Autodesk Inventor part; units mm, degrees
ref_plane "YZ Plane" through (0, 0, 0) normal (1, 0, 0) x (0, 1, 0)
ref_plane "XZ Plane" through (0, 0, 0) normal (0, 1, 0) x (-1, 0, 0)
ref_plane "XY Plane" through (0, 0, 0) normal (0, 0, 1) x (1, 0, 0)
sketch "Skizze1" plane through (0, 0, 0) normal (0, 0, 1) x (1, 0, 0)
  line L0 (-4.5, 3.25) -> (-4.5, 2.25)
  arc A0 (-3.564, 1.602) -> (-4.5, 2.25) centre (-4.5, 1.25) ccw
  line L1 (-3.564, 1.602) -> (-3.2351, 1.602)
  line L2 (-3.2351, 1.602) -> (-3.2351, 0.898)
  line L3 (-3.2351, 0.898) -> (-3.564, 0.898)
  arc A1 (-4.5, 0.25) -> (-3.564, 0.898) centre (-4.5, 1.25) ccw
  line L4 (-4.5, 0.25) -> (-4.5, -3.25)
  line L5 (-4.5, -3.25) -> (4.5, -3.25)
  line L6 (4.5, -3.25) -> (4.5, 0.25)
  arc A2 (3.564, 0.898) -> (4.5, 0.25) centre (4.5, 1.25) ccw
  line L7 (3.564, 0.898) -> (3.2351, 0.898)
  line L8 (3.2351, 0.898) -> (3.2351, 1.602)
  line L9 (3.2351, 1.602) -> (3.564, 1.602)
  arc A3 (4.5, 2.25) -> (3.564, 1.602) centre (4.5, 1.25) ccw
  line L10 (4.5, 2.25) -> (4.5, 3.25)
  line L11 (4.5, 3.25) -> (-4.5, 3.25)
  line L12 (4.575, -3.325) -> (-4.575, -3.325)
  line L13 (-4.575, -3.325) -> (-4.575, 0.328)
  arc A4 (-4.575, 0.328) -> (-3.6174, 0.973) centre (-4.5, 1.25) ccw
  line L14 (-3.6174, 0.973) -> (-3.3101, 0.973)
  line L15 (-3.3101, 0.973) -> (-3.3101, 1.527)
  line L16 (-3.3101, 1.527) -> (-3.6174, 1.527)
  arc A5 (-3.6174, 1.527) -> (-4.575, 2.172) centre (-4.5, 1.25) ccw
  line L17 (-4.575, 2.172) -> (-4.575, 3.325)
  line L18 (-4.575, 3.325) -> (4.575, 3.325)
  line L19 (4.575, 3.325) -> (4.575, 2.172)
  arc A6 (4.575, 2.172) -> (3.6174, 1.527) centre (4.5, 1.25) ccw
  line L20 (3.6174, 1.527) -> (3.3101, 1.527)
  line L21 (3.3101, 1.527) -> (3.3101, 0.973)
  line L22 (3.3101, 0.973) -> (3.6174, 0.973)
  arc A7 (3.6174, 0.973) -> (4.575, 0.328) centre (4.5, 1.25) ccw
  line L23 (4.575, 0.328) -> (4.575, -3.325)
  circle A8 centre (-15.1, -13.35) radius 3.5
  line L24 (-20.2, -17.25) -> (-22.2, -15.25)
  line L25 (-20.2, -17.25) -> (9.8, -17.25)
  line L26 (9.8, -17.25) -> (9.8, 6.75)
  line L27 (-11.8, 6.75) -> (9.8, 6.75)
  line L28 (-11.8, 11.75) -> (-11.8, 6.75)
  line L29 (-20.2, 11.75) -> (-11.8, 11.75)
  line L30 (-22.2, 9.75) -> (-20.2, 11.75)
  line L31 (-22.2, -15.25) -> (-22.2, 9.75)
  line L32 (-11.8, 6.75) -> (-9.8, 6.75)
  line L33 (-9.8, 6.75) -> (-9.8, 11.75)
  line L34 (-9.8, 11.75) -> (-11.8, 11.75)
  line L35 (-11.8, 11.75) -> (-11.8, 6.75)
  line L36 (9.8, 11.75) -> (-20.2, 11.75)
  circle A9 centre (-15.1, -13.35) radius 1.1
  line L37 (-22.2, -15.25) -> (-20.2, -17.25)
  line L38 (-22.2, -15.25) -> (-22.2, 9.75)
  line L39 (-20.2, 11.75) -> (-22.2, 9.75)
  line L40 (9.8, 11.75) -> (-20.2, 11.75)
  line L41 (9.8, -17.25) -> (9.8, 11.75)
  line L42 (9.8, -17.25) -> (-20.2, -17.25)
  line L43 (-10, 6.75) -> (10, 6.75)
  line L44 (10, 6.75) -> (10, -6.75)
  line L45 (10, -6.75) -> (-10, -6.75)
  line L46 (-10, -6.75) -> (-10, 6.75)
  line L47 (-10, 6.75) -> (10, -6.75) construction
  line L48 (10, 6.75) -> (-10, -6.75) construction
  line L49 (10, 6.75) -> (-10, 6.75)
  line L50 (-10, 6.75) -> (-10, 11.75)
  line L51 (-10, 11.75) -> (10, 11.75)
  line L52 (10, 11.75) -> (10, 6.75)
  line L53 (-4.575, 0.328) -> (-4.575, 2.172)
  line L54 (4.575, 0.328) -> (4.575, 2.172)
  line L55 (9.8, 11.75) -> (-20.2, 11.75)
  point P0 (0, 0)
  point P1 (4.5, -1.5)
  point P2 (4.575, -1.4985)
  dimension "d0" = 0.075
  dimension "d1" = 20
  dimension "d2" = 13.5
extrude "Extrusion1" add sketch "Skizze1" along normal blind 25 contours L45 L46 L27 L26 | L26 L43 L44 L45 | L27 L33 L36 L41 | L41 L51 L52 L43 | L27 L50 L34 L33
sketch "Skizze2" plane through (-10, 11.75, 0) normal (0, 1, 0) x (1, 0, 0)
  line L0 (20, 0) -> (0, 0)
  line L1 (0, 0) -> (0, -25)
  line L2 (20, -25) -> (0, -25)
  line L3 (20, 0) -> (20, -25)
  line L4 (10, -12.6) -> (10, 75.6)
  point P0 (10, 0)
  point P1 (10, -3)
  dimension "d5" = 3
hole "Bohrung1" at (0, 11.75, 3) direction (0, -1, 0) diameter 2.8 end through all
pattern_linear "Rechteckige Anordnung1" count 4 spacing 6 along (0, 0, 1) of "Bohrung1"
chamfer "Fasen1" distance 2 angle 45 4 edges at (-10, 2.5, 0) (-10, 2.5, 25) (10, 2.5, 0) (10, 2.5, 25)
sketch "Skizze3" plane through (0, 0, 25) normal (0, 0, 1) x (1, 0, 0)
  line L0 (-5, -18.15) -> (-5, -21.15)
  line L1 (-22.9, -3.25) -> (-19.9, -3.25)
  circle A0 centre (-15.1, -13.35) radius 1.4224
  line L2 (-5, -5.55) -> (-5, -8.55)
  arc A1 (-5, -5.55) -> (-7.3, -3.25) centre (-7.3, -5.55) ccw
  line L3 (-10.3, -3.25) -> (-7.3, -3.25)
  line L4 (-25.2, -23.45) -> (-5, -23.45)
  line L5 (-5, -23.45) -> (-5, -3.25)
  line L6 (-5, -3.25) -> (-25.2, -3.25)
  line L7 (-25.2, -3.25) -> (-25.2, -23.45)
  line L8 (-25.2, -23.45) -> (-5, -3.25) construction
  line L9 (-5, -23.45) -> (-25.2, -3.25) construction
  line L10 (-10.3, -3.1) -> (-7.3, -3.1)
  arc A2 (-4.85, -5.55) -> (-7.3, -3.1) centre (-7.3, -5.55) ccw
  line L11 (-4.85, -5.55) -> (-4.85, -8.55)
  line L12 (-4.85, -3.1) -> (-4.85, -23.6)
  line L13 (-4.85, -23.6) -> (-25.35, -23.6)
  line L14 (-25.35, -23.6) -> (-25.35, -3.1)
  line L15 (-25.35, -3.1) -> (-4.85, -3.1)
  point P0 (0, 0)
  dimension "d19" = 0.15
extrude "Extrusion2" cut sketch "Skizze3" against normal blind 25 contours L5 L2 A2 L11 L12 L13 L14 L15 L10 L6 L3 L1 L7 L4 L0 | L0 L5 L4 L7 L6 L1 L3 A1 L2 | A1 L6 A2 L5
fillet "Rundung1" radius 2 2 edges at (-4.85, -6.75, 12.5) (-10, -3.1, 12.5)
properties part number "OT2-Gripper_block"
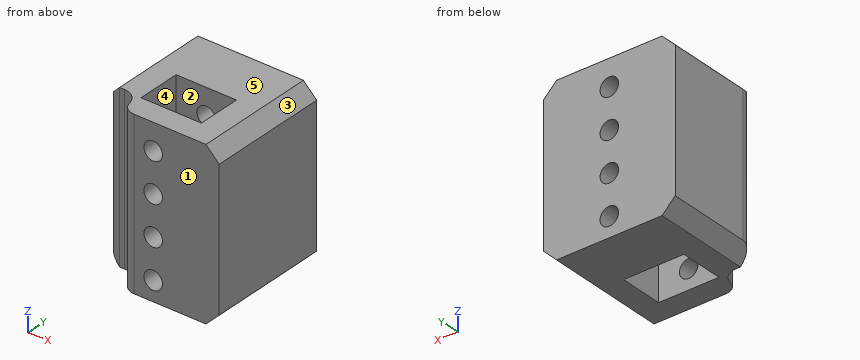
CAD build for the part. Positions are in the model's coordinates, mm. Face numbers are marked on the shaded views. A direction names the side the tool comes from. Round coordinates to 2 decimals unless told otherwise and drop trailing zeros. Loops run counter-clockwise (first coordinate to the right, second up) from the corner with the lowest first, then second, coordinate; pieces in that order, holes last. Notation, with made-up numbers: M -40,-6 L -15,-6 A31 ccw -15,33 Z; hole C 34,25.25 d11. An arc over 180 degrees is marked long. Return JSON: item names as keys, results as strings. Group by question number.
(1) Saw through at B-B, the plane y = 4.25. List the corners of the cut face in (x, z).
(2) Saw through at A-A, the plane x = 1.75. List the corners of the cut face in (y, z) (3 decimals).
(3) Mould opens along Y. For the marked faces 1, 2 and 3 say: +Y half, -Y half, draft (parallel to the pull), parting line (faces both ways), or undercut.
(4) Drop a flat-ended pin along its axis: P1, Ø1, axis at x = 0.5, z = 21.5, coming from the -Y side. Give the stop position or say it passes through.
(5) Wall check: probe 1 along Z at (x, y) = (0, -4.15); probe 2 along X at (y, z) = (-1.25, 18) (3 decimals); probe 3 along Y at (x, z) = (0.5, 1.25) (3 decimals). Give the ranges that are in metal, low to high. Write a range as [from, to].
(6) Saw through at D-D, the plane x = -6.25. List the corners of the cut face in (y, z), and give its area (3 significant figures).
(7) Saw through at C-C, the plane y = -1.75. List the corners of the cut face in (x, z) (3 decimals), and give its area (3 significant figures).
(8) Tool access for the marked faces 4 and 5: list every direction of +Z, -Z, +X, -X, +Y, -Y with a clear straight run to the whole face (end or side of a thin tool).
Answer list:
{
 "1": {"outline": "M -10,2 L -8,0 L 8,0 L 10,2 L 10,23 L 8,25 L -8,25 L -10,23 Z; hole C 0,3 d2.8; hole C 0,9 d2.8; hole C 0,15 d2.8; hole C 0,21 d2.8"},
 "2": {"outline": "M -6.75,0 L -3.325,0 L -3.325,25 L -6.75,25 Z; M 3.325,0 L 11.75,0 L 11.75,25 L 3.325,25 Z"},
 "3": {"face 1": "-Y half", "face 2": "undercut", "face 3": "draft"},
 "4": {"P1": "through"},
 "5": {"probe 1": "[0, 1.6], [4.4, 7.6], [10.4, 13.6], [16.4, 19.6], [22.4, 25]", "probe 2": "[-9.994, -4.575], [4.575, 10]", "probe 3": "[-6.75, -3.325], [3.325, 11.75]"},
 "6": {"outline": "M -3.34,0 L 11.75,0 L 11.75,25 L -3.34,25 Z", "area": "377 mm2"},
 "7": {"outline": "M -9.891,1.891 L -8,0 L -4.575,0 L -4.575,25 L -8,25 L -9.891,23.109 Z; M 4.575,0 L 8,0 L 10,2 L 10,23 L 8,25 L 4.575,25 Z", "area": "261 mm2"},
 "8": {"face 4": "+Z, -Z", "face 5": "+Z, +X, -X, +Y, -Y"}
}
